Can you work these out from the model? Positions are in its coordinate system, mm. A direction names the side the tool comes from. Round coordinates to 2 decimals unless told otherwise and drop trailing zeros. Loops run counter-clockwise (first coordinate to the right, second up) from the corner with the lowest first, then second, coordinate; pieces in that order, holes last. Notation, with made-up numbers: (42.5, 88) -> (99.5, 88) arc R26 ccw to (99.5, 112) -> close; hole circle Ø9 at (2.5, 55.25). An arc over 180 degrees is marked (long way). Write item = value, one per line.
from build123d import *

# Parameters (mm, degrees)
F1_DEPTH = 10
F3_DEPTH = 10
F5_DEPTH = 10


with BuildPart() as f1:
    # F0 (on Top) → F1 (new body)
    with BuildSketch(Plane.XY):
        with BuildLine():
            Line((0, 50), (0, 0))
            Line((0, 0), (20, 0))
            ThreePointArc((20, 0), (27.071068, 2.928932), (30, 10))
            Line((30, 10), (30, 30))
            Line((30, 30), (50, 30))
            ThreePointArc((50, 30), (57.071068, 32.928932), (60, 40))
            Line((60, 40), (60, 50))
            Line((60, 50), (0, 50))
        make_face()
    extrude(amount=F1_DEPTH)

    # F2 (on face) → F3 (join)
    with BuildSketch(Plane(origin=(0, 50, 0), x_dir=(-1, 0, 0), z_dir=(0, 1, 0))):
        with BuildLine():
            Line((-60, 10), (0, 10))
            Line((0, 10), (0, 30))
            Line((0, 30), (-20, 30))
            Line((-20, 30), (-20, 20))
            Line((-20, 20), (-50, 20))
            Line((-50, 20), (-50, 50))
            ThreePointArc((-50, 50), (-57.071068, 47.071068), (-60, 40))
            Line((-60, 40), (-60, 10))
        make_face()
    extrude(amount=-F3_DEPTH)

    # F4 (on face) → F5 (join)
    with BuildSketch(Plane(origin=(0, 0, 0), x_dir=(0, -1, 0), z_dir=(-1, 0, 0))):
        Polygon((0, 10), (-40, 30), (-40, 10), align=None)
    extrude(amount=-F5_DEPTH)


solid = f1.part
1. Suppose I cut it at D-D, the plane z = 38. List the corners of the cut face in (x, y) for me, and give its area (3 significant figures).
Entries:
outline = (50, 40) -> (60, 40) -> (60, 50) -> (50, 50) -> close
area = 100 mm²
2. Suppose I cut it at C-C, the plane z = 3.5. List the corners of the cut face in (x, y) for me, and give its area (3 significant figures).
Entries:
outline = (0, 0) -> (20, 0) arc R10 ccw to (30, 10) -> (30, 30) -> (50, 30) arc R10 ccw to (60, 40) -> (60, 50) -> (0, 50) -> close
area = 2,060 mm²
3. I'm going to push flat-ended pins straight in: pin 1 (2 mm diameter, centred on x = 23, y = 9, fed in from +Z); pin 2 (22 mm diameter, centred on y = 12, z = 16, fed in from +X); pin 3 (20 mm diameter, centred on x = 40.5, z = 22.5, fed in from -Y). Where does each tip first touch, or does it pass through?
Entries:
pin_1 = 10
pin_2 = 30
pin_3 = 40
4. We'd pull the mould along X, two halves only. Please class faces 6 (the flat face through (41, 40, 17)), 7 (the cylindrical face through (56.99, 32.85, 4.93)), 8 (the flat face through (0, 31, 12)), 9 (the flat face through (50, 45, 35)): released by +X, released by -X, zero draft, split by the parting line, or undercut.
Entries:
face_6 = zero draft
face_7 = released by +X
face_8 = released by -X
face_9 = undercut
5. Suppose I cut it at A-A, the plane z = 16. List the corners of the cut face in (x, y) for me.
Entries:
outline = (0, 12) -> (10, 12) -> (10, 40) -> (60, 40) -> (60, 50) -> (0, 50) -> close
6. For faces 1 (the flat face through (10, 45, 30)), 2 (the flat face through (40, 30, 5)), 3 (the flat face through (35, 45, 20)), 4 (the flat face through (10, 29, 16)), 5 (the flat face through (5, 20, 20)), which set-ups out of +Z, -Z, +X, -X, +Y, -Y let a thin tool reach every point of the face, with its end or its side?
Entries:
face_1 = +Z, -X, +Y, -Y
face_2 = +Z, -Z, +X, -Y
face_3 = +Z, +Y, -Y
face_4 = +Z, +X, -Y
face_5 = +Z, +X, -X, -Y
7. Suppose I cut it at B-B, the plane y = 19. List the corners of the cut face in (x, z) for me.
Entries:
outline = (0, 0) -> (30, 0) -> (30, 10) -> (10, 10) -> (10, 19.5) -> (0, 19.5) -> close
8. I need wall thicknesses on line 1 (X direction, y = 43.5, z = 28); line 2 (Y direction, x = 55, z = 42); line 3 (Z direction, x = 20, y = 39). Which ranges of each line are inside material? Lowest first, please. Write a range as [from, to].
Entries:
line_1 = [0, 20], [50, 60]
line_2 = [40, 50]
line_3 = [0, 10]
